from build123d import *

# Parameters (mm, degrees)
F2_R     = 4.7625
F3_DEPTH = 19.05


with BuildPart() as f3:
    # F2 (on Right) → F3 (new body)
    with BuildSketch(Plane.YZ):
        Polygon((-612.14, 228.6), (-497.84, 114.3), (-186.69, 114.3), (-109.22, 304.8), (-731.52, 304.8), (-731.52, 273.05), (-662.94, 228.6), align=None)
        with Locations((-601.345, 260.35)):
            Circle(F2_R, mode=Mode.SUBTRACT)
        with Locations((-712.47, 288.925)):
            Circle(F2_R, mode=Mode.SUBTRACT)
    extrude(amount=F3_DEPTH)


solid = f3.part
The model under review builds one solid part; all positions refer to its coordinate system, in mm. A direction names the side the tool comes from. Round coordinates to 2 decimals unless told otherwise and drop trailing zeros. Loops run counter-clockwise (first coordinate to the right, second up) from the corner with the lowest first, then second, coordinate; pieces in that order, holes last. Notation, with made-up numbers: M -28.5,45 L 20.5,45 A22 cw 20.5,76 Z; hole C 42.25,-35.5 d11. An arc over 180 degrees is marked long. Answer as CSV lines item,"result".
1. We need section A-A (x = 14). Count the separate pieces of the cut face and the enclosed holes in it, plus the area to 3 significant figures.
Outcome:
separate pieces,"1"
enclosed holes,"2"
area,"89,300 mm2"
2. For faces 1 (the face through (9, -344, 114.3)), 2 (the face through (9, -638, 228.6)), list the 3-axis set-ups (+Z, -Z, +X, -X, +Y, -Y) from which the entire face can be reached by the end or side of a thin tool; tool diameter is ignored.
Outcome:
face 1,"-Z, +X, -X, +Y, -Y"
face 2,"-Z, +X, -X, -Y"
3. To check wall thickness, follow L1, parallel to Z at x = 15, y = -712.47; L2, parallel to Y at x = 9.5, z = 260.35; L3, parallel to Z at x = 8.75, y = -652. State the ranges of each line that lie inside material, in increasing order. Write a range as [from, to].
Outcome:
L1,"z = [260.7, 284.16], [293.69, 304.8]"
L2,"y = [-711.93, -606.11], [-596.58, -127.3]"
L3,"z = [228.6, 304.8]"
4. We need section B-B (y = -559). Give the boundary of the cut face in (x, z).
Outcome:
outline,"M 0,175.46 L 19.05,175.46 L 19.05,304.8 L 0,304.8 Z"
5. Insertion check: pin 1 Ø6 at (x, z) = (12, 209.5) entering from -Y; pin 2 Ø3 at (y, z) = (-241, 164) entering from -X; pin 3 Ø8.5 at (y, z) = (-601.345, 260.35) entering from -X; pin 4 Ø5 at (x, z) = (12, 271) entering from +Y. Each pin has a flat end and moves straight along its axis. Give the tip position at first contact, or say it passes through.
Outcome:
pin 1,"stops at y = -596.04"
pin 2,"stops at x = 0"
pin 3,"passes through"
pin 4,"stops at y = -121.95"
6. We need section C-C (z = 203). Give the boundary of the cut face in (x, y), plus the area to 3 significant figures.
Outcome:
outline,"M 0,-586.54 L 19.05,-586.54 L 19.05,-150.62 L 0,-150.62 Z"
area,"8,300 mm2"
